The figure shows three views and two pictorial views of one solid part (mm, origin at its lowest corner). Answer the questions. Round coordinates to 2 decimals unless told otherwise and drop trailing zeros. Write each loop counter-clockwise with the first axis right and the second up, starting at its lowest first coordinate (ties: lowest second). Pieces come first, ordered by that corner, then holes.
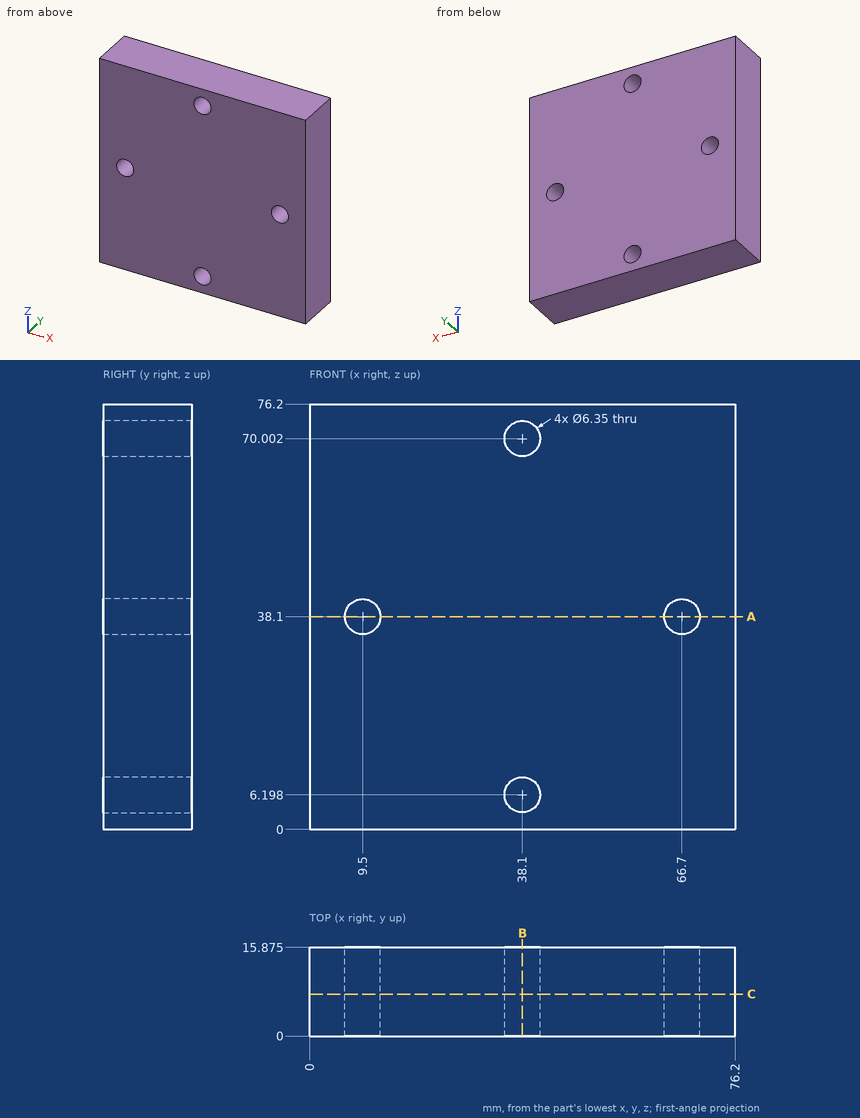
Q1. Section A-A (z = 38.1) is taken. Determine the outline of the cut face in (x, y) (1 decimal).
Verdict:
outline: (0, 0) - (6.3, 0) - (6.3, 15.9) - (0, 15.9) - close; (12.7, 0) - (63.5, 0) - (63.5, 15.9) - (12.7, 15.9) - close; (69.9, 0) - (76.2, 0) - (76.2, 15.9) - (69.9, 15.9) - close
Q2. Straight lines are drawn through the part: probe 1 along X at (y, z) = (3, 38.1) (1 decimal); probe 2 along Z at (x, y) = (36, 1.25) (1 decimal); probe 3 along X at (y, z) = (2, 4). For each, find the intervals that lie inside material, in ascending order.
Verdict:
probe 1: x = 0 to 6.3, 12.7 to 63.5, 69.9 to 76.2
probe 2: z = 0 to 3.8, 8.6 to 67.6, 72.4 to 76.2
probe 3: x = 0 to 35.81, 40.39 to 76.2
Q3. Flat-ended cylindrical pins translate along their axes: pin 1 Ø12 at (x, z) = (62.5, 43) entering from -Y; pin 2 Ø4 at (x, z) = (9.5, 38.1) entering from +Y. Find the tip coordinate at first contact, or state that the pin passes through.
Verdict:
pin 1: stops at y = 0
pin 2: passes through
Q4. Section B-B (x = 38.1) is taken. Determine the outline of the cut face in (y, z) (1 decimal), then the cut area to 3 significant figures.
Verdict:
outline: (0, 0) - (15.9, 0) - (15.9, 3) - (0, 3) - close; (0, 9.4) - (15.9, 9.4) - (15.9, 66.8) - (0, 66.8) - close; (0, 73.2) - (15.9, 73.2) - (15.9, 76.2) - (0, 76.2) - close
area: 1,010 mm2
Q5. Section C-C (y = 7.5) is taken. State how many separate pieces and enclosed holes the cut face has, then the cut area to 3 significant figures.
Verdict:
separate pieces: 1
enclosed holes: 4
area: 5,680 mm2
